```python
from build123d import *

# Parameters (mm, degrees)
F0_W     = 47.344006598
F0_H     = 58.3720691502
F1_DEPTH = 128.4994799644
F2_R     = 6.9700197205
F4_DEPTH = 115.1127442718


with BuildPart() as f1:
    # F0 (on Front) → F1 (new body)
    with BuildSketch(Plane.XZ):
        with Locations((23.672003299, 29.1860345751)):
            Rectangle(F0_W, F0_H)
    extrude(amount=F1_DEPTH)

    # F2
    f2_edges = [f1.edges().sort_by_distance(p)[0] for p in [
        (23.672003, -128.49948, 58.372069),
        (47.344007, -64.24974, 58.372069),
        (0, -64.24974, 58.372069),
        (23.672003, 0, 58.372069),
        (47.344007, -128.49948, 29.186035),
        (0, -128.49948, 29.186035),
        (23.672003, -128.49948, 0),
        (47.344007, -64.24974, 0),
        (47.344007, 0, 29.186035),
        (0, 0, 29.186035),
        (23.672003, 0, 0),
        (0, -64.24974, 0),
    ]]
    fillet(f2_edges, radius=F2_R)

    # F3 (on face) → F4 (join)
    with BuildSketch(Plane.XY.offset(58.3720691502)):
        with BuildLine():
            Line((6.9700197205, -60.7335358806), (6.9700197205, -9.472435718))
            ThreePointArc((6.9700197205, -9.472435718), (-19.2179336437, -35.1029857993), (6.9700197205, -60.7335358806))
        make_face()
        with BuildLine():
            ThreePointArc((6.9700197205, -60.7335358806), (24.7402160172, -53.03468171), (32.0550306924, -35.1029857993))
            ThreePointArc((32.0550306924, -35.1029857993), (24.7402160172, -17.1712898886), (6.9700197205, -9.472435718))
            Line((6.9700197205, -9.472435718), (6.9700197205, -60.7335358806))
        make_face()
    extrude(amount=F4_DEPTH)


solid = f1.part
```
The listing builds one solid part. Answer for the finished solid, in the listing's coordinates (mm). A direction names the side the tool comes from. Give positions to 0.01 mm unless a question says otherwise; leave off trailing zeros. Loops run counter-clockwise (first coordinate to the right, second up) from the corner with the lowest first, then second, coordinate; pieces in that order, holes last. Notation, with made-up numbers: (-12.5, 83) - (-1.5, 83) arc R13 ccw to (-1.5, 92) - close; hole circle Ø2 at (30, -13). An arc over 180 degrees is marked (long way). Answer as CSV lines item,"result". Start each with the question number.
Item 1: Each of these flat-tipped pins is pushed along its axis until it touches: pin 1 (10 mm diameter, centred on x = 20.5, y = -88.5, fed in from +Z); pin 2 (12 mm diameter, centred on x = 6.5, z = 105, fed in from +Y); pin 3 (12 mm diameter, centred on x = -8, y = -51.5, fed in from -Z). Where does it stop, or does it pass through?
Item 2: A cutting plane is placed at B-B on y = -92. Determine the outline of the cut face in (x, z).
Item 3: A cutting plane is placed at A-A on x = 35.5. Determine the outline of the cut face in (y, z).
Item 4: For faces 4 (the face through (45.25, -65.05, 1.99)), 5 (the face through (0, -63, 29)), determine the directions among +Z, -Z, +X, -X, +Y, -Y from which every point of the face is accessible in a straight line to the end or side of a thin tool.
Item 5: A cutting plane is placed at D-D on x = 15. Determine the outline of the cut face in (y, z).
Item 6: The mould has two halves that part along Z. Classify faces 1 (the face through (1.99, -65.05, 56.28)), 2 (the face through (45.356, -65.052, 56.276)), 3 (the face through (23.906, -126.404, 1.988)): +Z half, -Z half, draft (parallel to the pull), parting line (faces both ways), or undercut.
Item 7: A cutting plane is placed at C-C on z = 156.5. Determine the outline of the cut face in (x, y).
Item 8: Find the intervals of material crossed by line 1 (Z direction, x = 18, y = -8.5); line 2 (Z direction, x = 41, y = -77); line 3 (X direction, y = -115.5, z = 44), in increasing order. Write a range as from..to.
Found:
1,pin 1,"stops at z = 58.37"
1,pin 2,"stops at y = -9.47"
1,pin 3,"stops at z = 58.37"
2,outline,"(0, 6.97) arc R6.97 ccw to (6.97, 0) - (40.37, 0) arc R6.97 ccw to (47.34, 6.97) - (47.34, 51.4) arc R6.97 ccw to (40.37, 58.37) - (6.97, 58.37) arc R6.97 ccw to (0, 51.4) - close"
3,outline,"(-128.5, 6.97) arc R6.97 ccw to (-121.53, 0) - (-6.97, 0) arc R6.97 ccw to (0, 6.97) - (0, 51.4) arc R6.97 ccw to (-6.97, 58.37) - (-121.53, 58.37) arc R6.97 ccw to (-128.5, 51.4) - close"
4,face 4,"-Z, +X, +Y, -Y"
4,face 5,"-Z, -X, +Y, -Y"
5,outline,"(-128.5, 6.97) arc R6.97 ccw to (-121.53, 0) - (-6.97, 0) arc R6.97 ccw to (0, 6.97) - (0, 51.4) arc R6.97 ccw to (-6.97, 58.37) - (-10.95, 58.37) - (-10.95, 173.48) - (-59.26, 173.48) - (-59.26, 58.37) - (-121.53, 58.37) arc R6.97 ccw to (-128.5, 51.4) - close"
6,face 1,"undercut"
6,face 2,"+Z half"
6,face 3,"-Z half"
7,outline,"circle Ø51.27 at (6.42, -35.1)"
8,line 1,"z = 0..58.37"
8,line 2,"z = 0.03..58.34"
8,line 3,"x = 0..47.34"
